Verification items for the finished model (mm, model axes). Face numbers are marked on the shaded views. Round coordinates to 2 decimals unless told otherwise and drop trailing zeros. Write each loop counter-clockwise with the first axis right and the second up, starting at its lowest first coordinate (ties: lowest second). Pieces come first, ordered by that corner, then holes. Notation, with made-up numbers: (-37, -32.5) - (-2, -32.5) arc R8 cw to (-2, -18.5) - close; hole circle Ø11 at (-21.75, 84). An arc over 180 degrees is marked (long way). Write each question's results on one line, items separated by ' | '.
```python
from build123d import *

# Parameters (mm, degrees)
BASE_EXTRUDE_DEPTH         = 20
SZKIC1_OUTSIDE_W           = 72.884
SZKIC1_OUTSIDE_H           = 66.542
SZKIC1_OUTSIDE_R           = 18.915964881
WYTNIJ_WYCI_GNI_CIE1_DEPTH = 3
WYTNIJ_WYCI_GNI_CIE1_DRAFT = -60
SZKIC2_OUTSIDE_W           = 72.884
SZKIC2_OUTSIDE_H           = 66.542
SZKIC2_OUTSIDE_R           = 19.068904069
WYTNIJ_WYCI_GNI_CIE2_DEPTH = 3
WYTNIJ_WYCI_GNI_CIE2_DRAFT = -60
OTW_R_GWINTOWANY_M241_D    = 21
SFAZOWANIE1_SIZE           = 1


with BuildPart() as part:
    # Sketch1 → Base-Extrude (new body)
    with BuildSketch(Plane.XY):
        Polygon((23.671361037, 0), (11.835680518, 20.5), (-11.835680518, 20.5), (-23.671361037, 0), (-11.835680518, -20.5), (11.835680518, -20.5), align=None)
    extrude(amount=BASE_EXTRUDE_DEPTH)


with BuildPart() as wytnij_wyci_gni_cie1_tool:
    # Szkic1 outside → Wytnij-wyciągnięcie1 (with draft: the straight prism first)
    with BuildSketch(Plane.XY.offset(20)):
        Rectangle(SZKIC1_OUTSIDE_W, SZKIC1_OUTSIDE_H)
        Circle(SZKIC1_OUTSIDE_R, mode=Mode.SUBTRACT)
    extrude(amount=-WYTNIJ_WYCI_GNI_CIE1_DEPTH)
    # Wytnij-wyciągnięcie1: the draft: its side faces are tilted about the plane it starts from
    wytnij_wyci_gni_cie1_sides = [wytnij_wyci_gni_cie1_tool.faces().sort_by_distance(p)[0] for p in [
        (0, -33.271, 18.5),
        (36.442, 0, 18.5),
        (0, 33.271, 18.5),
        (-36.442, 0, 18.5),
        (-18.915964881, 0, 18.5),
    ]]
    draft(wytnij_wyci_gni_cie1_sides, Plane.XY.offset(20), WYTNIJ_WYCI_GNI_CIE1_DRAFT)


with BuildPart() as part_1:
    add(part.part)

    # Wytnij-wyciągnięcie1: cut by wytnij_wyci_gni_cie1_tool
    add(wytnij_wyci_gni_cie1_tool.part, mode=Mode.SUBTRACT)


with BuildPart() as wytnij_wyci_gni_cie2_tool:
    # Szkic2 outside → Wytnij-wyciągnięcie2 (with draft: the straight prism first)
    with BuildSketch(Plane(origin=(0, 0, 0), x_dir=(-1, 0, 0), z_dir=(0, 0, -1))):
        Rectangle(SZKIC2_OUTSIDE_W, SZKIC2_OUTSIDE_H)
        Circle(SZKIC2_OUTSIDE_R, mode=Mode.SUBTRACT)
    extrude(amount=-WYTNIJ_WYCI_GNI_CIE2_DEPTH)
    # Wytnij-wyciągnięcie2: the draft: its side faces are tilted about the plane it starts from
    wytnij_wyci_gni_cie2_sides = [wytnij_wyci_gni_cie2_tool.faces().sort_by_distance(p)[0] for p in [
        (0, -33.271, 1.5),
        (-36.442, 0, 1.5),
        (0, 33.271, 1.5),
        (36.442, 0, 1.5),
        (19.068904069, 0, 1.5),
    ]]
    draft(wytnij_wyci_gni_cie2_sides, Plane(origin=(0, 0, 0), x_dir=(-1, 0, 0), z_dir=(0, 0, -1)), WYTNIJ_WYCI_GNI_CIE2_DRAFT)


with BuildPart() as part_2:
    add(part_1.part)

    # Wytnij-wyciągnięcie2: cut by wytnij_wyci_gni_cie2_tool
    add(wytnij_wyci_gni_cie2_tool.part, mode=Mode.SUBTRACT)

    # Otwór gwintowany M241 (through all)
    with Locations(Plane(origin=(0, 0, 0), x_dir=(-1, 0, 0), z_dir=(0, 0, -1))):
        with Locations((0, 0)):
            Hole(OTW_R_GWINTOWANY_M241_D / 2)

    # Sfazowanie1
    sfazowanie1_edges = [part_2.edges().sort_by_distance(p)[0] for p in [
        (-10.5, 0, 0),
        (-10.5, 0, 20),
    ]]
    chamfer(sfazowanie1_edges, length=SFAZOWANIE1_SIZE)


solid = part_2.part
```
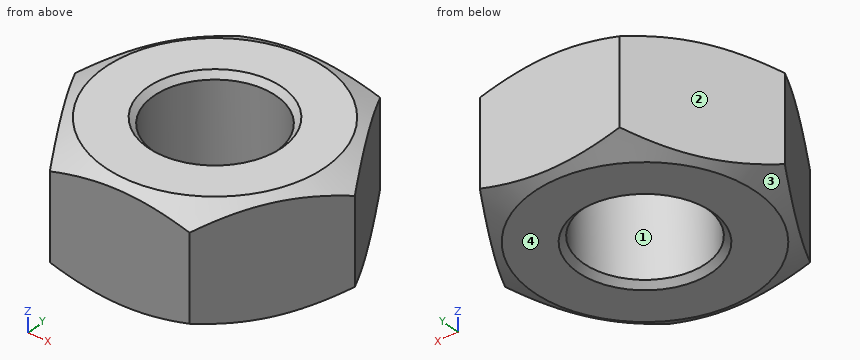
(1) Mould release check, pull along Y, two halves, no side actions. Record for the marked faces 1, 2, 3 and 4: released by +Y, released by -Y, zero draft, split by the parting line, or undercut.
Answer:
face 1: undercut | face 2: released by +Y | face 3: split by the parting line | face 4: zero draft
(2) Go/stop test with flat-tipped pins: pin 1 Ø19 at (x, y) = (0, 0) entering from +Z; pin 2 Ø5 at (x, z) = (15.5, 8) entering from +Y; pin 3 Ø12 at (y, z) = (-13.5, 14.5) entering from -X; pin 4 Ø4 at (y, z) = (3, 2) entering from +X. Record where each tip stops, or that it passes through.
Answer:
pin 1: through | pin 2: y = 18.48 | pin 3: x = -19.34 | pin 4: x = 23.08
(3) Section check C-C (z = 1.75). Record the cut outline in (x, y), plus the area to 3 significant figures.
Answer:
outline: (-21.88, -3.1) - (-13.63, -17.4) arc R22.1 ccw to (-8.26, -20.5) - (8.26, -20.5) arc R22.1 ccw to (13.63, -17.4) - (21.88, -3.1) arc R22.1 ccw to (21.88, 3.1) - (13.63, 17.4) arc R22.1 ccw to (8.26, 20.5) - (-8.26, 20.5) arc R22.1 ccw to (-13.63, 17.4) - (-21.88, 3.1) arc R22.1 ccw to start; hole circle Ø21 at (0, 0) | area: 1,080 mm2
(4) Thickness scan on L1, parallel to Y at x = 0, z = 7; L2, parallel to X at y = 9, z = 11.75; L3, parallel to Y at x = -13.5, z = 18.5. Record the ranges inside material, lowest first.
Answer:
L1: -20.5 to -10.5, 10.5 to 20.5 | L2: -18.48 to -5.41, 5.41 to 18.48 | L3: -16.75 to 16.75
(5) Section check B-B (x = 0). Record the cut outline in (y, z), plus the area to 3 significant figures.
Answer:
outline: (-20.5, 0.83) - (-19.07, 0) - (-11.5, 0) - (-10.5, 1) - (-10.5, 19) - (-11.5, 20) - (-18.92, 20) - (-20.5, 19.09) - close; (10.5, 1) - (11.5, 0) - (19.07, 0) - (20.5, 0.83) - (20.5, 19.09) - (18.92, 20) - (11.5, 20) - (10.5, 19) - close | area: 395 mm2
(6) Section check A-A (z = 13.25). Record the cut outline in (x, y), plus the area to 3 significant figures.
Answer:
outline: (-23.67, 0) - (-11.84, -20.5) - (11.84, -20.5) - (23.67, 0) - (11.84, 20.5) - (-11.84, 20.5) - close; hole circle Ø21 at (0, 0) | area: 1,110 mm2
